```python
from build123d import *

# Parameters (mm, degrees)
SKETCH6_R           = 0.225
EXTRUDE2_DEPTH      = 6.5
CUT_EXTRUDE1_DEPTH  = 8.611175993
BOSS_EXTRUDE1_START = 0.25
SKETCH10_R          = 0.8
BOSS_EXTRUDE1_DEPTH = 0.25
FILLET1_R           = 0.2
FILLET2_R           = 0.1
SKETCH6_3_R         = 0.5
SKETCH6_3_R_2       = 0.225
BOSS_EXTRUDE2_DEPTH = 0.35
FILLET4_R           = 0.1
FILLET5_R           = 0.1
FILLET6_R           = 0.1
FILLET7_R           = 0.1
FILLET8_R           = 0.1


with BuildPart() as part:
    # Sketch4 → Revolve2 (revolve)
    with BuildSketch(Plane.XY, mode=Mode.PRIVATE) as revolve2_sk:
        with BuildLine():
            Line((0, 0), (0, 0.7))
            Line((0, 0.7), (-0.65, 0.7))
            Line((-0.65, 0.7), (-0.65, 0.8))
            Line((-0.65, 0.8), (-0.95, 0.8))
            Line((-0.95, 0.8), (-0.95, 1.775))
            Line((-0.95, 1.775), (0.8, 1.775))
            ThreePointArc((0.8, 1.775), (0.976776695, 1.848223305), (1.05, 2.025))
            Line((1.05, 2.025), (1.05, 2.1))
            Line((1.05, 2.1), (1.35, 2.1))
            Line((1.35, 2.1), (1.35, 2.8))
            Line((1.35, 2.8), (2.55, 2.8))
            Line((2.55, 2.8), (2.55, 0))
            Line((2.55, 0), (0, 0))
        make_face()
    revolve(revolve2_sk.sketch.rotate(Axis((-2.49171246, 0, 0), (1, 0, 0)), 90), axis=Axis((-2.49171246, 0, 0), (1, 0, 0)))

    # Sketch6 → Extrude2 (add)
    with BuildSketch(Plane(origin=(2.55, 0, 0), x_dir=(0, 0, -1), z_dir=(1, 0, 0))):
        with Locations(Location((0, -1, 0), (0, 0, 180))):
            Circle(SKETCH6_R)
        with Locations(Location((-1, 0, 0), (0, 0, 180))):
            Circle(SKETCH6_R)
        with Locations(Location((1, 0, 0), (0, 0, 180))):
            Circle(SKETCH6_R)
    extrude(amount=EXTRUDE2_DEPTH)

    # Sketch8 → Cut-Extrude1 (cut, through all)
    with BuildSketch(Plane(origin=(2.55, 0, 0), x_dir=(0, 0, -1), z_dir=(1, 0, 0))):
        with BuildLine():
            Line((-2.4, 0), (-2.774801575, 0.374801575))
            ThreePointArc((-2.774801575, 0.374801575), (-2.8, 0), (-2.774801575, -0.374801575))
            Line((-2.774801575, -0.374801575), (-2.4, 0))
        make_face()
        with BuildLine():
            Line((2.774801575, 0.374801575), (2.4, 0))
            Line((2.4, 0), (2.774801575, -0.374801575))
            ThreePointArc((2.774801575, -0.374801575), (2.793693291, -0.187823841), (2.8, 0))
            ThreePointArc((2.8, 0), (2.793693291, 0.187823841), (2.774801575, 0.374801575))
        make_face()
        with BuildLine():
            ThreePointArc((-0.5, -2.754995463), (0, -2.8), (0.5, -2.754995463))
            Line((0.5, -2.754995463), (0.5, -2.4))
            Line((0.5, -2.4), (-0.5, -2.4))
            Line((-0.5, -2.4), (-0.5, -2.754995463))
        make_face()
    extrude(amount=-CUT_EXTRUDE1_DEPTH, mode=Mode.SUBTRACT)

    # Sketch10 → Boss-Extrude1 (add)
    with BuildSketch(Plane.ZY.offset(0.65).offset(BOSS_EXTRUDE1_START)):
        Circle(SKETCH10_R)
    extrude(amount=-BOSS_EXTRUDE1_DEPTH)

    # Fillet1
    fillet1_edges = [part.edges().sort_by_distance(p)[0] for p in [
        (-0.95, 0, -1.775),
    ]]
    fillet(fillet1_edges, radius=FILLET1_R)

    # Fillet2
    fillet2_edges = [part.edges().sort_by_distance(p)[0] for p in [
        (1.35, 2.8, 0),
        (1.35, -1.934576937, -2.02420653),
        (1.35, -1.934576937, 2.02420653),
    ]]
    fillet(fillet2_edges, radius=FILLET2_R)

    # Sketch6_3 → Boss-Extrude2 (add)
    with BuildSketch(Plane(origin=(2.55, 0, 0), x_dir=(0, 0, -1), z_dir=(1, 0, 0))):
        with Locations(Location((0, -1, 0), (0, 0, 180))):
            Circle(SKETCH6_3_R)
        with Locations((0, -1)):
            Circle(SKETCH6_3_R_2, mode=Mode.SUBTRACT)
    extrude(amount=BOSS_EXTRUDE2_DEPTH)

    # Fillet4
    fillet4_edges = [part.edges().sort_by_distance(p)[0] for p in [
        (1.95, -2.4, 0.5),
    ]]
    fillet(fillet4_edges, radius=FILLET4_R)

    # Fillet5
    fillet5_edges = [part.edges().sort_by_distance(p)[0] for p in [
        (1.95, -2.4, -0.5),
    ]]
    fillet(fillet5_edges, radius=FILLET5_R)

    # Fillet6
    fillet6_edges = [part.edges().sort_by_distance(p)[0] for p in [
        (1.378931181, -2.724856522, -0.5),
        (1.378985991, -2.724912772, 0.5),
        (1.35, -2.429289322, 0.470710678),
        (1.35, -2.4, 0),
        (1.35, -2.429289322, -0.470710678),
        (2, -2.754995463, -0.5),
        (2, -2.754995463, 0.5),
        (1.35, -2.576649916, 0.5),
        (1.35, -2.576649916, -0.5),
    ]]
    fillet(fillet6_edges, radius=FILLET6_R)

    # Fillet7
    fillet7_edges = [part.edges().sort_by_distance(p)[0] for p in [
        (1.95, 0, 2.4),
    ]]
    fillet(fillet7_edges, radius=FILLET7_R)

    # Fillet8
    fillet8_edges = [part.edges().sort_by_distance(p)[0] for p in [
        (1.95, 0, -2.4),
    ]]
    fillet(fillet8_edges, radius=FILLET8_R)


solid = part.part
```
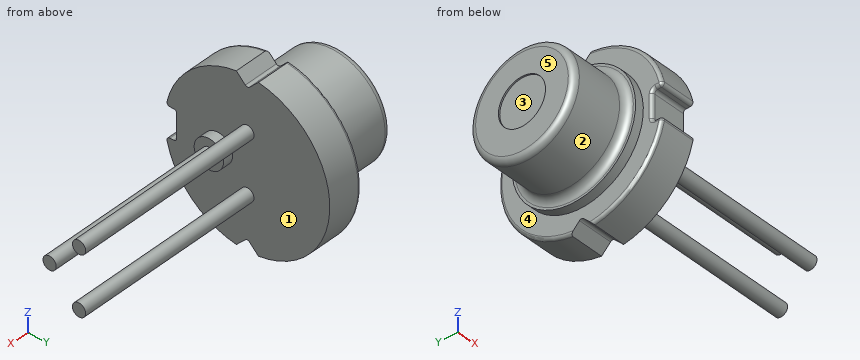
CAD build for the part. Positions are in the model's coordinates, mm. Face numbers are marked on the shaded views. A direction names the side the tool comes from. Round coordinates to 2 decimals unless told otherwise and drop trailing zeros. Order: outer loops, then holes, each group sorted by start corner. A loop starts at its lowest first (then second) coordinate and runs counter-clockwise, first axis right, second up. Notation, with made-up numbers: (-22.75, 80) - (-14.75, 80) arc R25 cw to (-14.75, 97) - close; hole circle Ø4 at (66.5, -14.5). An arc over 180 degrees is marked (long way). Use CSV: the item, a comma, the result in double quotes. Start each with the question number.
1) Saw through at C-C (x = 4.75). List the corners of the cut face in (y, z) (3 decimals).
2) Pin check, flat tips, straight feed: pin 1 Ø0.5 at (y, z) = (0, -0.5) entering from -X; pin 2 Ø0.7 at (y, z) = (0.5, 0.5) entering from +X. Stop position of each tip, or through.
3) Wall check: L1, parallel to Y at x = -0.2, z = 0 (3 decimals); L2, parallel to X at y = 0.4, z = 0.15; L3, parallel to X at y = -1.25, z = -1.55. Give the ranges that are in metal, low to high. Write a range as [from, to].
4) Two-plate mould, pull along Y, no slides. Class the marked faces 1, 2 and 3: pulls with the +Y half, pulls with the -Y half, needs draft (parallel to the pull), parting line crosses it, or undercut.
5) Saw through at B-B (x = 2). List the corners of the cut face in (y, z).
6) Tool access for the marked faces 4 and 5: list every direction of +Z, -Z, +X, -X, +Y, -Y with a clear straight run to the whole face (end or side of a thin tool).
Values follow:
1,outline,"circle Ø0.45 at (-1, 0); circle Ø0.45 at (0, -1); circle Ø0.45 at (0, 1)"
2,pin 1,"stops at x = -0.9"
2,pin 2,"stops at x = 2.55"
3,L1,"y = [-1.775, -0.7], [0.7, 1.775]"
3,L2,"x = [-0.9, -0.65], [0, 2.55]"
3,L3,"x = [1.05, 2.55]"
4,face 1,"needs draft"
4,face 2,"parting line crosses it"
4,face 3,"undercut"
5,outline,"(-2.73, -0.62) arc R2.8 ccw to (-0.37, -2.77) - (-0.07, -2.47) arc R0.1 cw to (0.07, -2.47) - (0.37, -2.77) arc R2.8 ccw to (0.37, 2.77) - (0.07, 2.47) arc R0.1 cw to (-0.07, 2.47) - (-0.37, 2.77) arc R2.8 ccw to (-2.73, 0.62) arc R0.1 ccw to (-2.63, 0.5) - (-2.5, 0.5) arc R0.1 cw to (-2.4, 0.4) - (-2.4, -0.4) arc R0.1 cw to (-2.5, -0.5) - (-2.63, -0.5) arc R0.1 ccw to start"
6,face 4,"-X"
6,face 5,"+Z, -Z, -X, +Y, -Y"
